```python
from build123d import *

# Parameters (mm, degrees)
F0_W   = 5.2163470536
F0_H   = 1.59855932
F0_W_2 = 4.0384605527


with BuildPart() as f1:
    # F0 (on Front) → F1 (revolve)
    with BuildSketch(Plane.XZ):
        with Locations((2.6081735268, 53.0468784273)):
            Rectangle(F0_W, F0_H)
        Polygon((0, 50.6490394473), (0, 0), (13.7980775908, 0), (13.7980775908, 50.6490394473), (9.2548076063, 50.6490394473), (5.2163470536, 50.6490394473), align=None)
        with Locations((7.23557733, 51.4483191073)):
            Rectangle(F0_W_2, F0_H)
        with Locations((2.6081735268, 51.4483191073)):
            Rectangle(F0_W, F0_H)
    revolve(axis=Axis((0, 0, 25.3245197237), (0, 0, 1)))


solid = f1.part
```
The model under review builds one solid part; all positions refer to its coordinate system, in mm. A direction names the side the tool comes from. Give positions to 0.01 mm unless a question says otherwise; leave off trailing zeros. Write each loop counter-clockwise with the first axis right and the second up, starting at its lowest first coordinate (ties: lowest second). Pieces come first, ordered by that corner, then holes. Notation, with made-up numbers: M -21,12 L -1,12 A33 cw -1,41 Z; hole C -7,-23.5 d5. An arc over 180 degrees is marked long. Write each question's results on one line, items separated by ' | '. Start each with the question number.
1. For probe 1 along Z at (x, y) = (-6.75, 9.5); probe 2 along Z at (x, y) = (6.25, -5.75); probe 3 along Y at (x, z) = (0, 37.5), list the stretches that pass through material, from the lowest coordinate up. Write a range as [from, to].
2. Insertion check: pin 1 Ø10 at (x, z) = (-1, 14) entering from -Y; pin 2 Ø1 at (x, z) = (-4.5, 21.5) entering from -Y; pin 3 Ø6 at (y, z) = (9, 41) entering from +X; pin 4 Ø4 at (x, z) = (-10.5, 17) entering from +Y. Each pin has a flat end and moves straight along its axis. Give the tip position at first contact, or say it passes through.
3. Mouldability with a two-part tool opening along Y and no side actions: class faces 3 (the cylindrical face through (-2.99, -13.47, 25.68)), 4 (the flat face through (-4, -4, 52.248)) as released by +Y, released by -Y, zero draft, split by the parting line, or undercut.
4. We need section A-A (y = 0). Write out the cut boundary in (x, z), and give its area (3 significant figures).
5. We need section D-D (x = -7.5). Write out the cut boundary in (y, z).
6. For faces 1 (the flat face through (0, 0, 0)), 2 (the flat face through (9, -3, 50.649)), list the 3-axis set-ups (+Z, -Z, +X, -X, +Y, -Y) from which the entire face can be reached by the end or side of a thin tool; tool diameter is ignored.
7. We need section C-C (z = 17.5). Write out the cut boundary in (x, y), and give its area (3 significant figures).
Results found:
1) probe 1: z = [0, 50.65] | probe 2: z = [0, 52.25] | probe 3: y = [-13.8, 13.8]
2) pin 1: stops at y = -13.8 | pin 2: stops at y = -13.21 | pin 3: stops at x = 12.43 | pin 4: stops at y = 10.87
3) face 3: split by the parting line | face 4: zero draft
4) outline: M -13.8,0 L 13.8,0 L 13.8,50.65 L 9.25,50.65 L 9.25,52.25 L 5.22,52.25 L 5.22,53.85 L -5.22,53.85 L -5.22,52.25 L -9.25,52.25 L -9.25,50.65 L -13.8,50.65 Z | area: 1,440 mm^2
5) outline: M -11.58,0 L 11.58,0 L 11.58,50.65 L 5.42,50.65 L 5.42,52.25 L -5.42,52.25 L -5.42,50.65 L -11.58,50.65 Z
6) face 1: -Z, +X, -X, +Y, -Y | face 2: +Z
7) outline: C 0,0 d27.6 | area: 598 mm^2
